from build123d import *

# Parameters (mm, degrees)
F0_W           = 80
F0_H           = 70
F0_R           = 13
F1_DEPTH       = 45
F2_R           = 16
F3_DEPTH       = 15
F5_R           = 16.85
F6_DEPTH       = 1.3
F8_D           = 8
F8_DEPTH       = 36
F8_CBORE_D     = 8
F8_CBORE_DEPTH = 0
F8_TIP         = 2.4034424761


with BuildPart() as f1:
    # F0 (on Front) → F1 (new body)
    with BuildSketch(Plane.XZ):
        with Locations((40, 35)):
            Rectangle(F0_W, F0_H)
        with Locations((40, 40)):
            Circle(F0_R, mode=Mode.SUBTRACT)
    extrude(amount=F1_DEPTH)

    # F2 (on face) → F3 (cut)
    with BuildSketch(Plane.XZ.offset(45)):
        with Locations((40, 40)):
            Circle(F2_R)
    extrude(amount=-F3_DEPTH, mode=Mode.SUBTRACT)

    # F5 (on offset) → F6 (cut)
    with BuildSketch(Plane.XZ.offset(39)):
        with Locations((40, 40)):
            Circle(F5_R)
    extrude(amount=F6_DEPTH, mode=Mode.SUBTRACT)

    # F8
    with Locations(Plane(origin=(0, 0, 0), x_dir=(1, 0, 0), z_dir=(0, 0, -1))):
        with Locations((15, 22.5), (65, 22.5)):
            CounterBoreHole(F8_D / 2, F8_CBORE_D / 2, F8_CBORE_DEPTH, depth=F8_DEPTH)
            with Locations((0, 0, -(F8_DEPTH + F8_TIP / 2))):  # 118° drill point
                Cone(0, F8_D / 2, F8_TIP, mode=Mode.SUBTRACT)


solid = f1.part
The listing builds one solid part. Answer for the finished solid, in the listing's coordinates (mm). A direction names the side the tool comes from. Coordinates: 2 decimals unless noted, no trailing zeros. Loops run counter-clockwise (first coordinate to the right, second up) from the corner with the lowest first, then second, coordinate; pieces in that order, holes last.
1) Find section C-C on z = 7. Write down the section's boundary in (x, y).
2) Flat-ended cylindrical pins translate along their axes: pin 1 Ø2 at (y, z) = (-33.5, 37.5) entering from -X; pin 2 Ø5 at (x, z) = (28.5, 40.5) entering from -Y. Find the tip coordinate at first contact, or state that the pin passes through.
3) Find the intervals of material crossed by L1, parallel to X at y = -22.5, z = 9; L2, parallel to Y at x = 15, z = 11.5; L3, parallel to X at y = -20.25, z = 40, in increasing order.
4) Determine the mould class of faces 1 (the face through (39, -22, 0)), 2 (the face through (39, -45, 20)), 3 (the face through (27.013, -14.79, 40.572)) for opening direction Z: pulls with the +Z half, pulls with the -Z half, needs draft (parallel to the pull), parting line crosses it, or undercut.
5) Find section A-A on x = 40. Write down the section's boundary in (y, z), then the cut area to 3 significant figures.
6) A tool of negligible diameter and unlimited length cuts with its end or side. For faces 4 (the face through (61.185, -23.701, 18.252)), 5 (the face through (24.015, -34.563, 40.703)), 6 (the face through (55, -39, 34)), from which of +Z, -Z, +X, -X, +Y, -Y can it reach the whole face along a straight path? Write none if from no direction.
7) Find section B-B on z = 40. Write down the section's boundary in (x, y).
8) Find section D-D on y = -31.5. Write down the section's boundary in (x, z), then the cut area to 3 significant figures.
Values:
1. outline: (0, -45) - (80, -45) - (80, 0) - (0, 0) - close; hole circle Ø8 at (15, -22.5); hole circle Ø8 at (65, -22.5)
2. pin 1: stops at x = 0
2. pin 2: stops at y = -30
3. L1: x = 0 to 11, 19 to 61, 69 to 80
3. L2: y = -45 to -26.5, -18.5 to 0
3. L3: x = 0 to 27, 53 to 80
4. face 1: pulls with the -Z half
4. face 2: needs draft
4. face 3: undercut
5. outline: (-45, 0) - (0, 0) - (0, 27) - (-30, 27) - (-30, 24) - (-39, 24) - (-39, 23.15) - (-40.3, 23.15) - (-40.3, 24) - (-45, 24) - close; (-45, 56) - (-40.3, 56) - (-40.3, 56.85) - (-39, 56.85) - (-39, 56) - (-30, 56) - (-30, 53) - (0, 53) - (0, 70) - (-45, 70) - close
5. area: 1,890 mm2
6. face 4: -Z
6. face 5: -Y
6. face 6: none
7. outline: (0, -45) - (24, -45) - (24, -40.3) - (23.15, -40.3) - (23.15, -39) - (24, -39) - (24, -30) - (27, -30) - (27, 0) - (0, 0) - close; (53, -30) - (56, -30) - (56, -39) - (56.85, -39) - (56.85, -40.3) - (56, -40.3) - (56, -45) - (80, -45) - (80, 0) - (53, 0) - close
8. outline: (0, 0) - (80, 0) - (80, 70) - (0, 70) - close; hole circle Ø32 at (40, 40)
8. area: 4,800 mm2
